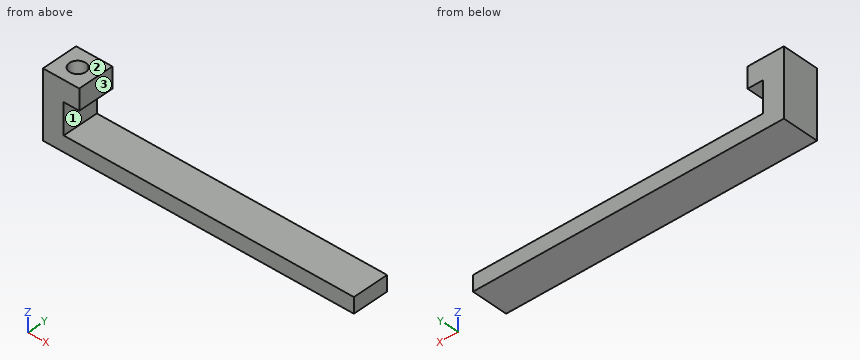
Autodesk Fusion 360 part; units mm, degrees
sketch "Sketch1" plane through (0, 0, 0) normal (0, 0, 1) x (1, 0, 0)
  line L0 (0, 0) -> (76.2, 0)
  line L1 (76.2, 0) -> (76.2, 8.89)
  line L2 (76.2, 8.89) -> (0, 8.89)
  line L3 (0, 8.89) -> (0, 0)
  dimension "d1" = 76.2
  dimension "d2" = 8.89
extrude "Extrude1" add sketch "Sketch1" along normal blind 3.81
sketch "Sketch2" plane through (0, 0, 3.81) normal (0, 0, 1) x (-1, 0, 0)
  line L0 (0, -8.89) -> (0, 0)
  line L1 (0, 0) -> (-76.2, 0)
  line L2 (-76.2, 0) -> (-76.2, -8.89)
  line L3 (-76.2, -8.89) -> (0, -8.89)
  line L4 (0, 0) -> (-5.08, 0)
  line L5 (-5.08, 0) -> (-5.08, -8.89)
  line L6 (-5.08, -8.89) -> (0, -8.89)
  line L7 (0, -8.89) -> (0, 0)
  dimension "d5" = 5.08
extrude "Extrude2" add sketch "Sketch2" along normal blind 7.62 contours L0 L1 L3 L4 L5 L6 L7
sketch "Sketch3" plane through (0, 0, 11.43) normal (0, 0, 1) x (-1, 0, 0)
  line L0 (0, -8.89) -> (0, 0)
  line L1 (0, 0) -> (-5.08, 0)
  line L2 (-5.08, 0) -> (-5.08, -8.89)
  line L3 (-5.08, -8.89) -> (0, -8.89)
  line L4 (0, 0) -> (-8.89, 0)
  line L5 (-8.89, 0) -> (-8.89, -8.89)
  line L6 (-8.89, -8.89) -> (0, -8.89)
  line L7 (0, -8.89) -> (0, 0)
  dimension "d8" = 8.89
extrude "Extrude3" add sketch "Sketch3" along normal blind 5.08
hole "Hole1" at (4.445, 4.445, 16.51) direction (0, 0, -1) diameter 4 depth 4 tip angle 180
Geometry: final body of the model. Coordinates: model frame, mm. Face numbers are marked on the shaded views. Give positions to 0.01 mm unless a question says otherwise; leave off trailing zeros. Write each loop counter-clockwise with the first axis right and the second up, starting at its lowest first coordinate (ties: lowest second). Pieces come first, ordered by that corner, then holes.
1. Section query A-A, the plane y = 8. Return loops of the section in (x, z), then the cut area to 3 significant figures.
2. Pin query (flat end, axial travel): P1, Ø1.5, axis at y = 2, z = 7.5, coming from the -X side; P2, Ø1.5, axis at y = 5, z = 14.5, coming from the +X side; P3, Ø2, axis at x = 4, y = 4, coming from the +Z side; P4, Ø4, axis at y = 2.5, z = 7.5, coming from the +X side. Return the tip coordinate at first contact, or that it passes through.
3. Section query C-C, the plane z = 14.25. Return loops of the section in (x, y) (3 decimals).
4. Section query B-B, the plane z = 9.5. Return loops of the section in (x, y).
5. Draft query along Z for the marked faces 1, 2 and 3. Return one class per face: released by +Z, released by -Z, zero draft, split by the parting line, or undercut.
6. Section query D-D, the plane x = 27. Return loops of the section in (y, z).
7. Line query: probe 1 along Z at (x, y) = (6, 2); probe 2 along X at (y, z) = (4.5, 15.5); probe 3 along X at (y, z) = (5, 10). Output: solid intervals per line, ascending.
Computed:
1. outline: (0, 0) - (76.2, 0) - (76.2, 3.81) - (5.08, 3.81) - (5.08, 11.43) - (8.89, 11.43) - (8.89, 16.51) - (0, 16.51) - close
1. area: 374 mm2
2. P1: stops at x = 0
2. P2: stops at x = 8.89
2. P3: stops at z = 12.51
2. P4: stops at x = 5.08
3. outline: (0, 0) - (8.89, 0) - (8.89, 8.89) - (0, 8.89) - close; hole circle Ø4 at (4.445, 4.445)
4. outline: (0, 0) - (5.08, 0) - (5.08, 8.89) - (0, 8.89) - close
5. face 1: undercut
5. face 2: released by +Z
5. face 3: zero draft
6. outline: (0, 0) - (8.89, 0) - (8.89, 3.81) - (0, 3.81) - close
7. probe 1: z = 0 to 3.81, 11.43 to 16.51
7. probe 2: x = 0 to 2.45, 6.44 to 8.89
7. probe 3: x = 0 to 5.08
